from build123d import *

# Parameters (mm, degrees)
SKETCH1_W                = 10
SKETCH1_H                = 15
BOSS_EXTRUDE1_DEPTH      = 73
F_6_0_6_DIAMETER_HOLE1_D = 6
F_6_0_6_DIAMETER_HOLE2_D = 6
M4X0_7_TAPPED_HOLE1_D    = 3.3


with BuildPart() as part:
    # Sketch1 → Boss-Extrude1 (new body)
    with BuildSketch(Plane.XY):
        Rectangle(SKETCH1_W, SKETCH1_H)
    extrude(amount=-BOSS_EXTRUDE1_DEPTH)

    # Ø6.0 (6) Diameter Hole1 (through all)
    with Locations(Plane(origin=(5, 0, 0), x_dir=(0, 0, -1), z_dir=(1, 0, 0))):
        with Locations((9, 0), (64, 0)):
            Hole(F_6_0_6_DIAMETER_HOLE1_D / 2)

    # Ø6.0 (6) Diameter Hole2 (through all)
    with Locations(Plane(origin=(5, 0, 0), x_dir=(0, 0, -1), z_dir=(1, 0, 0))):
        with Locations((30, 1.6)):
            Hole(F_6_0_6_DIAMETER_HOLE2_D / 2)

    # M4x0.7 Tapped Hole1 (through all)
    with Locations(Plane(origin=(0, 7.5, 0), x_dir=(1, 0, 0), z_dir=(0, 1, 0))):
        with Locations((0, 30)):
            Hole(M4X0_7_TAPPED_HOLE1_D / 2)


solid = part.part
Geometry: final body of the model. Coordinates: model frame, mm. Round coordinates to 2 decimals unless told otherwise and drop trailing zeros. Order: outer loops, then holes, each group sorted by start corner. A loop starts at its lowest first (then second) coordinate and runs counter-clockwise, first axis right, second up. Notation, with made-up numbers: (63, 29) -> (73, 29) arc R23 ccw to (73, 40) -> close; hole circle Ø10 at (48.5, -26). An arc over 180 degrees is marked (long way). Put each result on its own line as item: value. Start each with the question number.
Q1. Section A-A on z = -30. Return the cut outline in (x, y), and give its area (3 significant figures).
Q2. Section B-B on y = -2.25. Return the cut outline in (x, z), and give its area (3 significant figures).
Q3. Line query: probe 1 along Z at (x, y) = (0, 5.75); probe 2 along Z at (x, y) = (-1.25, 0.75); probe 3 along Z at (x, y) = (1.5, 3.75). Output: solid intervals per line, ascending.
Q4. First-contact query: pin 1 (2 mm diameter, centred on x = -2, y = -0.5, fed in from +Z). Flat tip, straight axial feed; report the tip coordinate or a pass-through.
Q5. Pull-direction query (Z, two-part tool) for faces 1 (the cylindrical face through (1.65, -4.25, -30.07)), 2 (the flat face through (5, 0, -36)), 3 (the flat face through (0, 0, 0)); classes: +Z half, -Z half, draft (parallel to the pull), parting line (faces both ways), or undercut.
Q6. Section D-D on z = -9. Return the cut outline in (x, y), and give its area (3 significant figures).
Q7. Section C-C on x = 0. Return the cut outline in (y, z).
Ans:
1. outline: (-5, -7.5) -> (-1.65, -7.5) -> (-1.65, -1.4) -> (-5, -1.4) -> close; (-5, 4.6) -> (-1.65, 4.6) -> (-1.65, 7.5) -> (-5, 7.5) -> close; (1.65, -7.5) -> (5, -7.5) -> (5, -1.4) -> (1.65, -1.4) -> close; (1.65, 4.6) -> (5, 4.6) -> (5, 7.5) -> (1.65, 7.5) -> close
1. area: 60.3 mm2
2. outline: (-5, -73) -> (5, -73) -> (5, -65.98) -> (-5, -65.98) -> close; (-5, -62.02) -> (5, -62.02) -> (5, -10.98) -> (-5, -10.98) -> close; (-5, -7.02) -> (5, -7.02) -> (5, 0) -> (-5, 0) -> close; hole circle Ø3.3 at (0, -30)
2. area: 642 mm2
3. probe 1: z = -73 to -31.65, -28.35 to 0
3. probe 2: z = -73 to -66.9, -61.1 to -32.88, -27.12 to -11.9, -6.1 to 0
3. probe 3: z = -73 to -32.09, -27.91 to 0
4. pin 1: stops at z = 0
5. face 1: undercut
5. face 2: draft
5. face 3: +Z half
6. outline: (-5, -7.5) -> (5, -7.5) -> (5, -3) -> (-5, -3) -> close; (-5, 3) -> (5, 3) -> (5, 7.5) -> (-5, 7.5) -> close
6. area: 90.0 mm2
7. outline: (-7.5, -73) -> (7.5, -73) -> (7.5, -31.65) -> (4.11, -31.65) arc R3 cw to (-0.91, -31.65) -> (-7.5, -31.65) -> close; (-7.5, -28.35) -> (-0.91, -28.35) arc R3 cw to (4.11, -28.35) -> (7.5, -28.35) -> (7.5, 0) -> (-7.5, 0) -> close; hole circle Ø6 at (0, -64); hole circle Ø6 at (0, -9)
